Autodesk Inventor part; units mm, degrees
ref_plane "YZ Plane" through (0, 0, 0) normal (1, 0, 0) x (0, 1, 0)
ref_plane "XZ Plane" through (0, 0, 0) normal (0, 1, 0) x (-1, 0, 0)
ref_plane "XY Plane" through (0, 0, 0) normal (0, 0, 1) x (1, 0, 0)
sketch "스케치1" plane through (0, 0, 0) normal (0, 0, 1) x (1, 0, 0)
  line L0 (9.6169, -10.809) -> (-9.6169, -10.809)
  line L1 (-9.6169, -10.809) -> (-9.6169, 10.809)
  line L2 (-9.6169, 10.809) -> (9.6169, 10.809)
  line L3 (9.6169, 10.809) -> (9.6169, -10.809)
  line L4 (9.6169, -10.809) -> (-9.6169, 10.809) construction
  line L5 (-9.6169, -10.809) -> (9.6169, 10.809) construction
  point P0 (0, 0)
extrude "돌출1" add sketch "스케치1" along normal blind 25
sketch "스케치2" plane through (-9.6169, 10.809, 0) normal (0, 1, 0) x (1, 0, 0)
  point P0 (9.6169, 0)
sketch "스케치3" plane through (0, 0, 25) normal (0, 0, 1) x (1, 0, 0)
  line L0 (9.6169, -10.809) -> (9.6169, 10.809)
  arc A0 (-6.8694, 10.809) -> (9.6169, -7.1319) centre (8.8168, 8.6782) ccw
  line L1 (-6.8694, 10.809) -> (9.6169, 10.809)
  point P0 (0, 0)
extrude "돌출2" cut sketch "스케치3" against normal blind 10
sketch "스케치4" plane through (0, 0, 0) normal (0, 0, -1) x (-1, 0, 0)
  line L0 (9.6169, 10.809) -> (9.6169, -10.809)
  line L1 (9.6169, 10.809) -> (-9.6169, -8.323)
  line L2 (-9.6169, 10.809) -> (-9.6169, -10.809)
  line L3 (-9.6169, -8.323) -> (-9.6169, 10.809)
  line L4 (9.6169, 10.809) -> (-9.6169, 10.809)
  line L5 (9.6169, 10.809) -> (-9.6169, 10.809)
  point P0 (0, 0)
sketch "스케치5" plane through (-9.6169, 10.809, 0) normal (0, 1, 0) x (1, 0, 0)
  line L0 (11.1073, -6.5575) -> (15.5096, -6.5575)
  line L1 (15.5096, -6.5575) -> (15.5096, -2.4763)
  line L2 (15.5096, -2.4763) -> (11.1073, -2.4763)
  line L3 (11.1073, -2.4763) -> (11.1073, -6.5575)
  line L4 (0, 0) -> (19.2339, 0)
  line L5 (0.0558, -2.4763) -> (5.1459, -2.4763)
  line L6 (5.1459, -2.4763) -> (5.1459, 0)
  line L7 (5.1459, 0) -> (0.0558, 0)
  line L8 (0.0558, 0) -> (0.0558, -2.4763)
  point P0 (9.6169, 0)
extrude "돌출3" cut sketch "스케치5" against normal blind 50 contours L3 L2 L1 L0
extrude "돌출4" cut sketch "스케치4" against normal blind 12
sketch "스케치6" plane through (-9.6169, -10.809, 25) normal (-1, 0, 0) x (0, 0, 1)
  line L0 (-25, 21.6179) -> (-13, 21.6179)
  line L1 (-25, 21.6179) -> (-21.9007, 21.6179)
  line L2 (-21.9007, 21.6179) -> (-21.9007, 17.0226)
  line L3 (-21.9007, 17.0226) -> (-25, 17.0226)
  line L4 (-25, 17.0226) -> (-25, 21.6179)
  point P0 (-25, 10.809)
extrude "돌출5" cut sketch "스케치6" against normal blind 12
properties part number "240510_3Dsketch08"
Source: CAD feature listing. Evaluate the final solid. Frame: model axes, mm. A direction names the side the tool comes from. Give positions to 0.01 mm unless a question says otherwise; leave off trailing zeros. Order: outer loops, then holes, each group sorted by start corner. A loop starts at its lowest first (then second) coordinate and runs counter-clockwise, first axis right, second up.
(1) Section query B-B (x = 2.75). Return the cut outline in (y, z).
(2) Material intervals for line 1 along Z through (x, y) = (4, -8.75); line 2 along Z through (x, y) = (3, -6); line 3 along Z through (x, y) = (-6, 6), sorted ascending.
(3) Section query C-C (z = 2). Return the cut outline in (x, y), plus the area to 3 significant figures.
(4) Section query A-A (z = 4.5). Return the cut outline in (x, y).
(5) Access query for faces 5 (the face through (4, -7, 2.476)), 6 (the face through (-7, 6.214, 2)), 7 (the face through (3, 4, 15)), 8 (the face through (2, 4, 12)). Directions: +Z, -Z, +X, -X, +Y, -Y. A direction counts if a zero-diameter tool reaches every point of the face in a straight line with its end or side. Return the directions, or none.
(6) Contact query for flat-ended pins moving along their axis: P1, Ø5, axis at x = 3.5, y = -7, coming from the -Z side; P2, Ø3.5, axis at x = 4, y = -4.5, coming from the +Z side; P3, Ø1.2, axis at y = -3, z = 4.5, coming from the +X side; P4, Ø4, axis at x = 0.5, z = 7.5, coming from the +Y side. Output: stop coordinate, or through.
(7) Section query D-D (y = -6.75). Return the cut outline in (x, z), plus the area to 3 significant figures.
(8) Pull-direction query (X, two-part tool) for faces 1 (the face through (-9.617, 0, 12)), 2 (the face through (1.49, -5, 4)), 3 (the face through (-8, 8, 3.099)), 4 (the face through (4, -7, 6.558)); classes: +X half, -X half, draft (parallel to the pull), parting line (faces both ways), or undercut.
Outcome:
1. outline: (-10.81, 0) - (-1.49, 0) - (-1.49, 2.48) - (-10.81, 2.48) - close; (-10.81, 6.56) - (-1.49, 6.56) - (-1.49, 12) - (10.81, 12) - (10.81, 15) - (-5.94, 15) - (-5.94, 25) - (-10.81, 25) - close
2. line 1: z = 0 to 2.48, 6.56 to 25
2. line 2: z = 0 to 2.48, 6.56 to 15
2. line 3: z = 0 to 15
3. outline: (-9.62, -10.81) - (9.62, -10.81) - (9.62, -8.32) - (-5, 6.21) - (-9.62, 6.21) - close
3. area: 221 mm2
4. outline: (-9.62, -10.81) - (1.49, -10.81) - (1.49, -0.24) - (-9.62, 10.81) - close; (5.89, -10.81) - (9.62, -10.81) - (9.62, -8.32) - (5.89, -4.62) - close
5. face 5: +Y, -Y
5. face 6: -Z, +X, -X, +Y
5. face 7: +Z, +X, +Y
5. face 8: -Z, +X, +Y
6. P1: stops at z = 0
6. P2: stops at z = 15
6. P3: stops at x = 1.49
6. P4: stops at y = 2.74
7. outline: (-9.62, 0) - (8.04, 0) - (8.04, 12) - (9.62, 12) - (9.62, 15) - (5.27, 15) - (5.27, 25) - (-9.62, 25) - close; hole (1.49, 2.48) - (5.89, 2.48) - (5.89, 6.56) - (1.49, 6.56) - close
7. area: 400 mm2
8. face 1: -X half
8. face 2: undercut
8. face 3: draft
8. face 4: undercut
